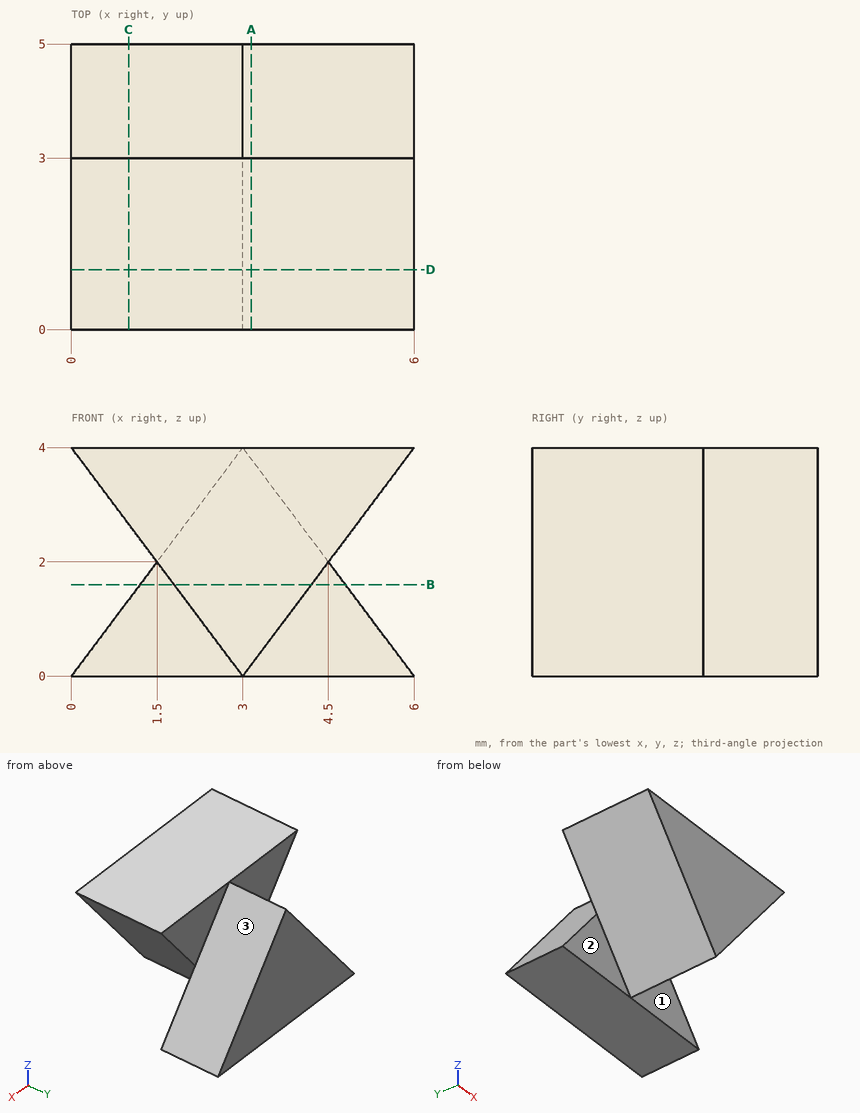
Input: dimensioned drawing with shaded views. Units: mm. Origin: part minimum x, y, z. A direction names the side the tool comes from. Coordinates: 2 decimals unless noted, no trailing zeros. Loops run counter-clockwise (first coordinate to the right, second up) from the corner with the lowest first, then second, coordinate; pieces in that order, holes last. Notation, with made-up numbers: (75.5, 79) -> (99.5, 79) arc R34 ccw to (99.5, 109) -> close; hole circle Ø3 at (26, 43.25). An arc over 180 degrees is marked (long way). One line per item, written item: value. Start each with the question number.
Q1. Set-up query: the marked faces 1, 2 and 3. Return all of +Z, -Z, +X, -X, +Y, -Y with unobstructed straight access to the full face (end or side cutting, diameter ignored); none if empty.
Q2. Section query B-B, the plane z = 1.6. Return the cut outline in (x, y).
Q3. Section query D-D, the plane y = 1.05. Return the cut outline in (x, z), and give its area (3 significant figures).
Q4. Section query C-C, the plane x = 1. Return the cut outline in (y, z), and give its area (3 significant figures).
Q5. Line query: line 1 along Y through (x, z) = (1.95, 3.3); line 2 along Y through (x, z) = (2.05, 0.75). Output: solid intervals per line, ascending.
Q6. Section query A-A, the plane x = 3.15. Return the cut outline in (y, z), and give its area (3 significant figures).
Results:
1. face 1: -Z, +X, -Y
1. face 2: -Z, -X, -Y
1. face 3: +Z, +X, +Y
2. outline: (1.2, 3) -> (1.8, 3) -> (1.8, 0) -> (4.2, 0) -> (4.2, 3) -> (4.8, 3) -> (4.8, 5) -> (1.2, 5) -> close
3. outline: (0, 4) -> (3, 0) -> (6, 4) -> close
3. area: 12.0 mm^2
4. outline: (0, 2.67) -> (3, 2.67) -> (3, 4) -> (0, 4) -> close; (3, 0) -> (5, 0) -> (5, 1.33) -> (3, 1.33) -> close
4. area: 6.67 mm^2
5. line 1: 0 to 3
5. line 2: 3 to 5
6. outline: (0, 0.2) -> (3, 0.2) -> (3, 0) -> (5, 0) -> (5, 3.8) -> (3, 3.8) -> (3, 4) -> (0, 4) -> close
6. area: 19.0 mm^2
